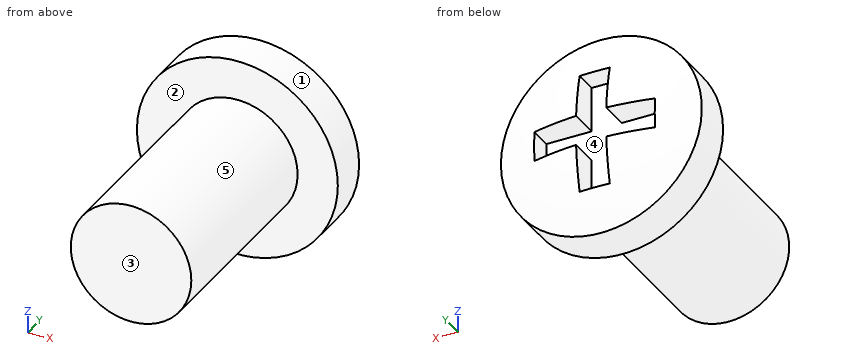
```python
from build123d import *

# Parameters (mm, degrees)
SKETCH1_R           = 1.5
BOSS_EXTRUDE1_DEPTH = 5
SKETCH2_R           = 2.5
BOSS_EXTRUDE2_DEPTH = 1
DOME1_FACE_RADIUS   = 2.5
DOME1_HEIGHT        = 0.5
SKETCH3_W           = 1.125
SKETCH3_H           = 0.75
SKETCH3_W_2         = 0.75
SKETCH3_H_2         = 1.125
CUT_EXTRUDE1_DEPTH  = 0.75


with BuildPart() as part:
    # Sketch1 → Boss-Extrude1 (new body)
    with BuildSketch(Plane(origin=(0, 0, 0), x_dir=(1, 0, 0), z_dir=(0, 1, 0))):
        Circle(SKETCH1_R)
    extrude(amount=BOSS_EXTRUDE1_DEPTH)

    # Sketch2 → Boss-Extrude2 (add)
    with BuildSketch(Plane(origin=(0, 5, 0), x_dir=(1, 0, 0), z_dir=(0, 1, 0))):
        Circle(SKETCH2_R)
    extrude(amount=BOSS_EXTRUDE2_DEPTH)

    # Dome1: a dome of height H over a round flat face of radius A is a cap of a sphere of radius (A * A + H * H) / (2 * H)
    dome1_r = (DOME1_FACE_RADIUS * DOME1_FACE_RADIUS + DOME1_HEIGHT * DOME1_HEIGHT) / (2 * DOME1_HEIGHT)
    dome1_base = Plane((0, 6, 0), z_dir=(0, 1, 0))
    with Locations(dome1_base.offset(DOME1_HEIGHT - dome1_r)):
        dome1_ball = Sphere(dome1_r, mode=Mode.PRIVATE)
    add(split(dome1_ball, bisect_by=dome1_base, keep=Keep.TOP, mode=Mode.PRIVATE))

    # Sketch3 → Cut-Extrude1 (cut)
    with BuildSketch(Plane(origin=(0, 6.5, 0), x_dir=(1, 0, 0), z_dir=(0, 1, 0))):
        with Locations((-0.9375, 0)):
            Rectangle(SKETCH3_W, SKETCH3_H)
        Rectangle(SKETCH3_W_2, SKETCH3_H)
        with Locations((0, 0.9375)):
            Rectangle(SKETCH3_W_2, SKETCH3_H_2)
        with Locations((0.9375, 0)):
            Rectangle(SKETCH3_W, SKETCH3_H)
        with Locations((0, -0.9375)):
            Rectangle(SKETCH3_W_2, SKETCH3_H_2)
    extrude(amount=-CUT_EXTRUDE1_DEPTH, mode=Mode.SUBTRACT)


solid = part.part
```
The model under review builds one solid part; all positions refer to its coordinate system, in mm. Face numbers are marked on the shaded views. A direction names the side the tool comes from. Coordinates: 2 decimals unless noted, no trailing zeros. Write each loop counter-clockwise with the first axis right and the second up, starting at its lowest first coordinate (ties: lowest second). Pieces come first, ordered by that corner, then holes.
1) The part is to be moulded in two halves that separate along Z. For the marked faces 3, 4 and 5, say which applies: pulls with the +Z half, pulls with the -Z half, needs draft (parallel to the pull), parting line crosses it, or undercut.
2) We need section D-D on x = -1.6. State the section outline as (y, z) points.
3) We need section A-A on x = 0. State the section outline as (y, z) points.
4) We need section C-C on y = 4. State the section outline as (x, z) points, then the cut area to 3 significant figures.
5) To check wall thickness, follow probe 1 along Y at (x, z) = (0.1, -0.75); probe 2 along Z at (x, y) = (-0.1, 5.25); probe 3 along X at (y, z) = (1.75, 0.65). State the ranges of each line that lie inside material, in increasing order.
6) Clearance check with flat-ended pins moving along their axes: pin 1 Ø2 at (x, z) = (-0.5, 0.5) entering from +Y; pin 2 Ø0.8 at (x, y) = (-1, 6) entering from +Z; pin 3 Ø1.5 at (x, y) = (-1, 5.5) entering from +Z; pin 4 Ø2 at (y, z) = (2, -1) entering from +X. State where each tip first meets the part, or that it passes through.
7) Machinability: for the marked faces 1 and 2, which of the approach directions +Z, -Z, +X, -X, +Y, -Y give a long, thin tool a straight path to every point of the face, cutting with its end or side? Answer none if there is none.
8) We need section B-B on z = 0. State the section outline as (x, y) points.
Answer list:
1. face 3: needs draft
1. face 4: undercut
1. face 5: parting line crosses it
2. outline: (5, -1.92) - (6, -1.92) arc R6.3 ccw to (6, 1.92) - (5, 1.92) - close
3. outline: (0, -1.5) - (5, -1.5) - (5, -2.5) - (6, -2.5) arc R6.5 ccw to (6.32, -1.5) - (5.75, -1.5) - (5.75, 1.5) - (6.32, 1.5) arc R6.5 ccw to (6, 2.5) - (5, 2.5) - (5, 1.5) - (0, 1.5) - close
4. outline: circle Ø3 at (0, 0)
4. area: 7.07 mm2
5. probe 1: y = 0 to 5.75
5. probe 2: z = -2.5 to 2.5
5. probe 3: x = -1.35 to 1.35
6. pin 1: stops at y = 6.48
6. pin 2: stops at z = 2.43
6. pin 3: stops at z = 2.49
6. pin 4: stops at x = 1.5
7. face 1: +Y, -Y
7. face 2: -Y
8. outline: (-2.5, 5) - (-1.5, 5) - (-1.5, 0) - (1.5, 0) - (1.5, 5) - (2.5, 5) - (2.5, 6) arc R6.5 ccw to (1.5, 6.32) - (1.5, 5.75) - (-1.5, 5.75) - (-1.5, 6.32) arc R6.5 ccw to (-2.5, 6) - close
